Study the drawing (mm; zero at the part's minimum x, y, z) and answer. Give positions to 0.01 mm unless a question says otherwise; leave off trailing zeros. Write each loop counter-clockwise with the first axis right and the second up, starting at its lowest first coordinate (ties: lowest second). Pieces come first, ordered by that corner, then holes. Notation, with made-up numbers: (-14, 36) -> (26, 36) arc R27 ccw to (26, 73) -> close; hole circle Ø6 at (9.25, 43). An arc over 180 degrees is marked (long way). One line per question, with ' | ' between items.
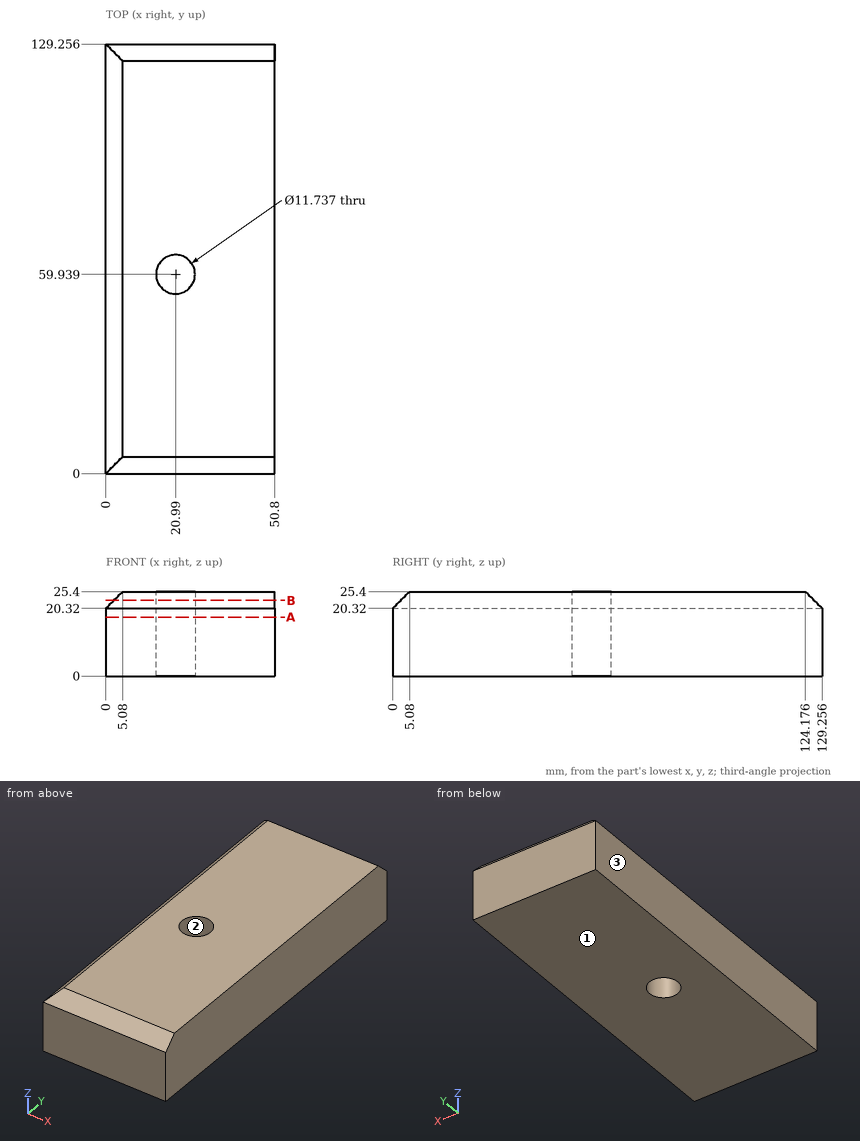
Item 1: Determine the mould class of the marked faces 1, 2 and 3 for opening direction X: pulls with the +X half, pulls with the -X half, needs draft (parallel to the pull), parting line crosses it, or undercut.
Answers below:
face 1: needs draft | face 2: undercut | face 3: pulls with the -X half
Item 2: Find section A-A (z = 17.75). Write down the section's boundary in (x, y).
Answers below:
outline: (0, 0) -> (50.8, 0) -> (50.8, 129.26) -> (0, 129.26) -> close; hole circle Ø11.74 at (20.99, 59.94)
Item 3: Find section B-B (z = 22.75). Write down the section's boundary in (x, y).
Answers below:
outline: (2.43, 2.43) -> (50.8, 2.43) -> (50.8, 126.83) -> (2.43, 126.83) -> close; hole circle Ø11.74 at (20.99, 59.94)
Item 4: A flat-ended cylindrical pin translates along its axis: pin 1 (13.5 mm diameter, centred on x = 20.99, y = 59.94, fed in from +Z). Find the tip coordinate at first contact, or state that the pin passes through.
Answers below:
pin 1: z = 25.4
Item 5: Consider line 1 (Y direction, x = 25.5, z = 23.5) (1 decimal); line 2 (X direction, y = 57.5, z = 19.5); line 3 (Y direction, x = 23.5, z = 10) (1 decimal). Determine where each line is inside the solid, lowest interval first. Write a range as [from, to].
Answers below:
line 1: [3.2, 56.2], [63.7, 126.1] | line 2: [0, 15.65], [26.33, 50.8] | line 3: [0, 54.6], [65.2, 129.3]
